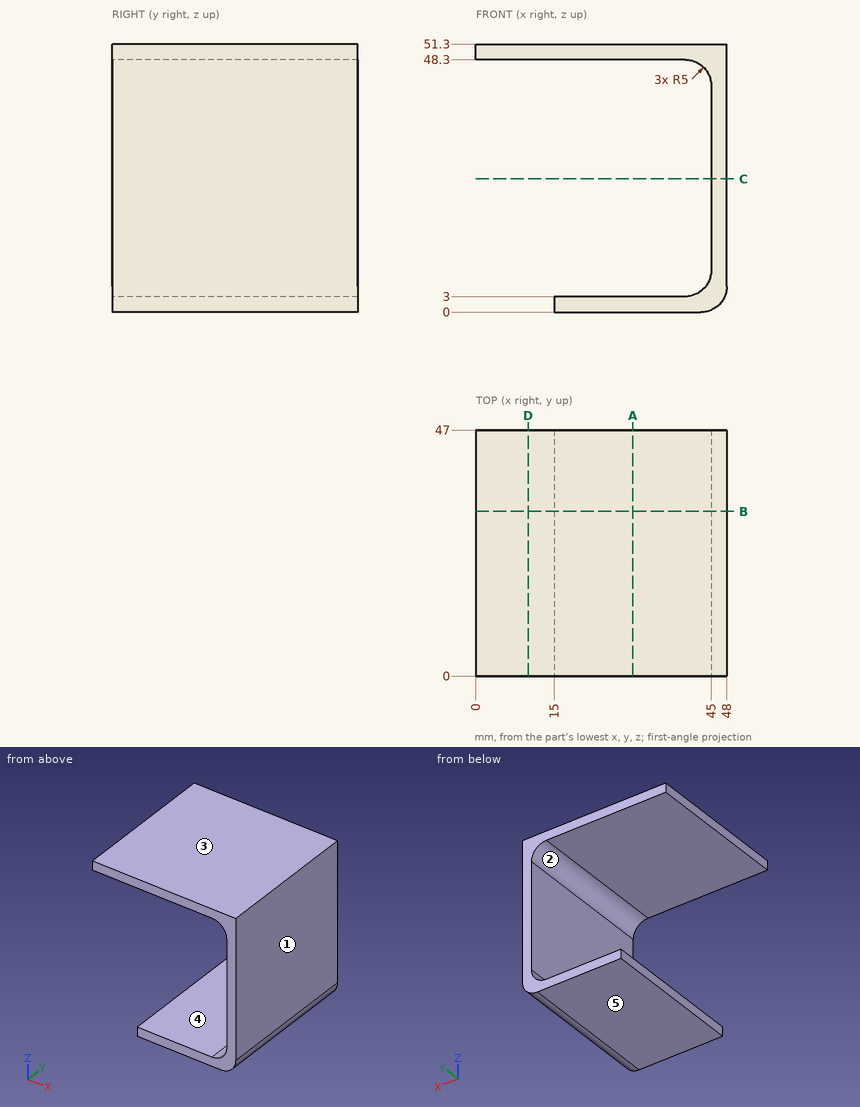
Design review of the part shown in the three views and the two pictorial views. Dimensions are in mm from the part's minimum x, y and z. A direction names the side the tool comes from. Give positions to 0.01 mm unless a question says otherwise; leave off trailing zeros. Loops run counter-clockwise (first coordinate to the right, second up) from the corner with the lowest first, then second, coordinate; pieces in that order, holes last. Notation, with made-up numbers: (69.5, -3.5) -> (126.5, -3.5) arc R23 ccw to (126.5, 11.5) -> close; hole circle Ø5 at (-21.75, -28). An arc over 180 degrees is marked (long way). Put each result on its own line as item: value. Start each with the question number.
1. We need section C-C on z = 25.5. State the section outline as (x, y) points, then the cut area to 3 significant figures.
2. We need section A-A on x = 30. State the section outline as (y, z) points.
3. Clearance check with flat-ended pins moving along their axes: P1, Ø12, axis at x = 14, y = 32.5, coming from the -Z side; P2, Ø2, axis at y = 35, z = 22, coming from the -X side; P3, Ø0.9, axis at y = 30.5, z = 1.5, coming from the -X side; P4, Ø10, axis at x = 23.5, z = 40.5, coming from the -Y side. State where each tip first meets the part, or that it passes through.
4. Mouldability with a two-part tool opening along Z and no side actions: class the marked faces 3, 4 and 5 as released by +Z, released by -Z, zero draft, split by the parting line, or undercut.
5. We need section B-B on y = 31.5. State the section outline as (x, z) points.
6. For the marked faces 1 and 2, list the 3-axis set-ups (+Z, -Z, +X, -X, +Y, -Y) from which the entire face can be reached by the end or side of a thin tool; tool diameter is ignored.
7. We need section D-D on x = 10. State the section outline as (y, z) points, then the cut area to 3 significant figures.
8. Wall thickness on probe 1 along Z at (x, y) = (30, 21); probe 2 along X at (y, z) = (10, 38); probe 3 along Z at (x, y) = (42.5, 24.5): over which ranges is each line inside the solid? List them lowest first.
Determined:
1. outline: (45, 0) -> (48, 0) -> (48, 47) -> (45, 47) -> close
1. area: 141 mm^2
2. outline: (0, 0) -> (47, 0) -> (47, 3) -> (0, 3) -> close; (0, 48.3) -> (47, 48.3) -> (47, 51.3) -> (0, 51.3) -> close
3. P1: z = 0
3. P2: x = 45
3. P3: x = 15
3. P4: through
4. face 3: released by +Z
4. face 4: undercut
4. face 5: released by -Z
5. outline: (0, 48.3) -> (40, 48.3) arc R5 cw to (45, 43.3) -> (45, 8) arc R5 cw to (40, 3) -> (15, 3) -> (15, 0) -> (43, 0) arc R5 ccw to (48, 5) -> (48, 51.3) -> (0, 51.3) -> close
6. face 1: +Z, -Z, +X, +Y, -Y
6. face 2: -X, +Y, -Y
7. outline: (0, 48.3) -> (47, 48.3) -> (47, 51.3) -> (0, 51.3) -> close
7. area: 141 mm^2
8. probe 1: 0 to 3, 48.3 to 51.3
8. probe 2: 45 to 48
8. probe 3: 0 to 3.67, 47.63 to 51.3
